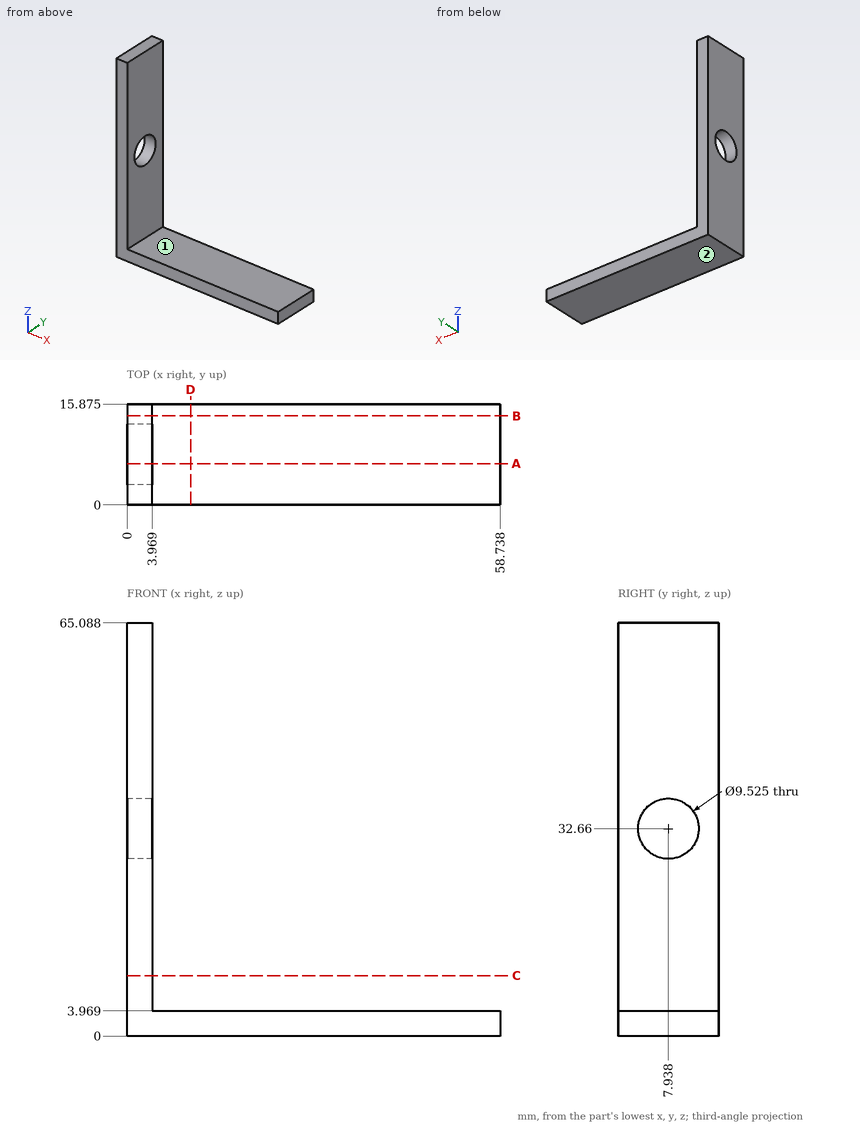
Study the drawing (mm; zero at the part's minimum x, y, z) and answer. A direction names the side the tool comes from. Coordinates: 2 decimals unless noted, no trailing zeros. Loops run counter-clockwise (first coordinate to the right, second up) from the corner with the lowest first, then second, coordinate; pieces in that order, holes last. Notation, with made-up numbers: M -11.5,32.5 L 39.5,32.5 A22 ccw 39.5,42.5 Z; hole C 5,-36 d9. An arc over 180 degrees is marked long. Answer as a JSON object with one key per item and string values. Group by question number.
Item 1: Section D-D (x = 10) is taken. Write down the section's boundary in (y, z) (1 decimal).
Item 2: Section C-C (z = 9.5) is taken. Write down the section's boundary in (x, y) (1 decimal).
Item 3: Each of these flat-tipped pins is pushed along its axis until it touches: P1, Ø5, axis at y = 9.5, z = 28.5, coming from the +X side; P2, Ø5, axis at x = 34.5, y = 10, coming from the +Z side; P3, Ø12, axis at x = 12.5, z = 33.5, coming from the -Y side. Where does it stop, or does it pass through?
Item 4: Section B-B (y = 14) is taken. Write down the section's boundary in (x, z).
Item 5: Consider L1, parallel to Y at x = 3, z = 33 (1 decimal); L2, parallel to Z at x = 54.5, y = 13. Determine where each line is inside the solid, lowest interval first.
Item 6: Which of the six approach directions +Z, -Z, +X, -X, +Y, -Y give full straight-line access (tool end or side, diameter ignored) to the marked faces 1 and 2?
Item 7: Section A-A (y = 6.5) is taken. Write down the section's boundary in (x, z).
Solved:
{
 "1": {"outline": "M 0,0 L 15.9,0 L 15.9,4 L 0,4 Z"},
 "2": {"outline": "M 0,0 L 4,0 L 4,15.9 L 0,15.9 Z"},
 "3": {"P1": "stops at x = 3.97", "P2": "stops at z = 3.97", "P3": "passes through"},
 "4": {"outline": "M 0,0 L 58.74,0 L 58.74,3.97 L 3.97,3.97 L 3.97,65.09 L 0,65.09 Z"},
 "5": {"L1": "y = 0 to 3.2, 12.7 to 15.9", "L2": "z = 0 to 3.97"},
 "6": {"face 1": "+Z, +X, +Y, -Y", "face 2": "-Z, +X, -X, +Y, -Y"},
 "7": {"outline": "M 0,0 L 58.74,0 L 58.74,3.97 L 3.97,3.97 L 3.97,28.12 L 0,28.12 Z; M 0,37.2 L 3.97,37.2 L 3.97,65.09 L 0,65.09 Z"}
}
